Part model, mm, in its own coordinate system. A direction names the side the tool comes from. Round coordinates to 2 decimals unless told otherwise and drop trailing zeros. Write each loop counter-clockwise with the first axis right and the second up, starting at its lowest first coordinate (ties: lowest second). Pieces come first, ordered by that corner, then holes. Notation, with made-up numbers: (25, 51) -> (47, 51) arc R21 ccw to (47, 79) -> close; hole circle Ø5 at (-38.5, 17.25). An arc over 180 degrees is marked (long way). Return JSON: item names as keys, results as strings. Group by question number.
Solid Edge part; units mm, degrees
sketch "Sketch1" plane through (0, 0, 0) normal (1, 0, 0) x (0, 1, 0)
  line L0 (42, -40) -> (42, 40)
  line L1 (42, 40) -> (-42, 40)
  line L2 (-42, 40) -> (-42, -40)
  line L3 (-42, -40) -> (42, -40)
extrude "Protrusion1" add sketch "Sketch1" along normal blind 2
sketch "Sketch2" plane through (0, 0, 0) normal (1, 0, 0) x (0, 1, 0)
  line L0 (-42, 38) -> (-25, 38)
  line L1 (-25, 38) -> (-25, 40)
  line L2 (-25, 40) -> (-42, 40)
  line L3 (-42, 40) -> (-42, 38)
  line L4 (-15, 38) -> (-5, 38)
  line L5 (-5, 38) -> (-5, 40)
  line L6 (-5, 40) -> (-15, 40)
  line L7 (-15, 40) -> (-15, 38)
  line L8 (5, 38) -> (15, 38)
  line L9 (15, 38) -> (15, 40)
  line L10 (15, 40) -> (5, 40)
  line L11 (5, 40) -> (5, 38)
  line L12 (25, 38) -> (42, 38)
  line L13 (42, 38) -> (42, 40)
  line L14 (42, 40) -> (25, 40)
  line L15 (25, 40) -> (25, 38)
  line L16 (40, 15) -> (40, 25)
  line L17 (40, 25) -> (38, 25)
  line L18 (38, 25) -> (38, 15)
  line L19 (38, 15) -> (40, 15)
  line L20 (38, 5) -> (38, -5)
  line L21 (38, -5) -> (40, -5)
  line L22 (40, -5) -> (40, 5)
  line L23 (40, 5) -> (38, 5)
  line L24 (38, -15) -> (38, -25)
  line L25 (38, -25) -> (40, -25)
  line L26 (40, -25) -> (40, -15)
  line L27 (40, -15) -> (38, -15)
  line L28 (42, -38) -> (25, -38)
  line L29 (25, -38) -> (25, -40)
  line L30 (25, -40) -> (42, -40)
  line L31 (42, -40) -> (42, -38)
  line L32 (15, -38) -> (5, -38)
  line L33 (5, -38) -> (5, -40)
  line L34 (5, -40) -> (15, -40)
  line L35 (15, -40) -> (15, -38)
  line L36 (-5, -38) -> (-15, -38)
  line L37 (-15, -38) -> (-15, -40)
  line L38 (-15, -40) -> (-5, -40)
  line L39 (-5, -40) -> (-5, -38)
  line L40 (-25, -38) -> (-42, -38)
  line L41 (-42, -38) -> (-42, -40)
  line L42 (-42, -40) -> (-25, -40)
  line L43 (-25, -40) -> (-25, -38)
  line L44 (-38, -25) -> (-38, -15)
  line L45 (-38, -15) -> (-40, -15)
  line L46 (-40, -15) -> (-40, -25)
  line L47 (-40, -25) -> (-38, -25)
  line L48 (-38, -5) -> (-38, 5)
  line L49 (-38, 5) -> (-40, 5)
  line L50 (-40, 5) -> (-40, -5)
  line L51 (-40, -5) -> (-38, -5)
  line L52 (-38, 15) -> (-38, 25)
  line L53 (-38, 25) -> (-40, 25)
  line L54 (-40, 25) -> (-40, 15)
  line L55 (-40, 15) -> (-38, 15)
extrude "ExtrudedCutout_29" cut sketch "Sketch2" along normal blind 2
sketch "Sketch3" plane through (0, 0, 0) normal (1, 0, 0) x (0, 1, 0)
  line L0 (30, 15) -> (-30, 15)
  line L1 (-30, 15) -> (-30, -15)
  line L2 (-30, -15) -> (30, -15)
  line L3 (30, -15) -> (30, 15)
extrude "ExtrudedCutout_30" cut sketch "Sketch3" along normal blind 2
sketch "Sketch4" plane through (0, 0, 0) normal (1, 0, 0) x (0, 1, 0)
  circle A0 centre (0, 20) radius 2.25
  circle A1 centre (0, -20) radius 2.25
extrude "ExtrudedCutout_31" cut sketch "Sketch4" along normal blind 2
fillet "Round_1" radius 1 4 edges at (1, -42, -38) (1, 42, -38) (1, 42, 38) (1, -42, 38)
properties material "Acrylic, high impact grade"
Item 1: Cut at D-D (y = 0). Write the cut outline in (x, z), then the cut area to 3 significant figures.
Item 2: Two-plate mould, pull along Z, no slides. Class faces 1 (the face through (1, 33, 38)), 2 (the face through (1, -20, -40)), 3 (the face through (1, 39, -15)), 4 (the face through (0.986, -0.488, 22.196)): released by +Z, released by -Z, zero draft, split by the parting line, or undercut.
Item 3: Which spindle directions (+Z, -Z, +X, -X, +Y, -Y) get a long thin tool onto all of the face, cutting with end or side? Do faces 5 (the face through (1, 5, 39)), 6 (the face through (1, 25, 39)), 7 (the face through (1, 10, -38)), 8 (the face through (1, 38, 20)). Say none if no direction does.
Item 4: Cut at C-C (z = 20). Write the cut outline in (x, y).
Item 5: Wall check: L1, parallel to Z at x = 0.55, y = 39.5; L2, parallel to Z at x = 1, y = 0; L3, parallel to Z at x = 1.95, y = -21.5. Give the ranges that are in metal, low to high.
Item 6: Cut at A-A (z = 9). Write the cut outline in (x, y), then the cut area to 3 significant figures.
Item 7: Cut at B-B (y = 20). Write the cut outline in (x, z).
Item 8: Flat gauge pins, fed straight in: P1, Ø0.6, axis at x = 1.5, z = 39.5, coming from the +Y side; P2, Ø1, axis at x = 0.5, y = -38.5, coming from the -Z side; P3, Ø8, axis at y = 30, z = -28.5, coming from the -X side; P4, Ø1, axis at x = 0.5, y = 39.5, coming from the +Z side. Where does each tip first touch, or does it go through?
Checks:
{
 "1": {"outline": "(0, -40) -> (2, -40) -> (2, -22.25) -> (0, -22.25) -> close; (0, -17.75) -> (2, -17.75) -> (2, -15) -> (0, -15) -> close; (0, 15) -> (2, 15) -> (2, 17.75) -> (0, 17.75) -> close; (0, 22.25) -> (2, 22.25) -> (2, 40) -> (0, 40) -> close", "area": "82.0 mm2"},
 "2": {"face 1": "released by +Z", "face 2": "released by -Z", "face 3": "undercut", "face 4": "undercut"},
 "3": {"face 5": "+Z, +X, -X", "face 6": "+Z, +X, -X, +Y", "face 7": "-Z, +X, -X", "face 8": "+X, -X"},
 "4": {"outline": "(0, -42) -> (2, -42) -> (2, -40) -> (0, -40) -> close; (0, -38) -> (2, -38) -> (2, -2.25) -> (0, -2.25) -> close; (0, 2.25) -> (2, 2.25) -> (2, 38) -> (0, 38) -> close; (0, 40) -> (2, 40) -> (2, 42) -> (0, 42) -> close"},
 "5": {"L1": "z = -38 to -25, -15 to -5, 5 to 15, 25 to 38", "L2": "z = -40 to -22.25, -17.75 to -15, 15 to 17.75, 22.25 to 40", "L3": "z = -40 to -15, 15 to 40"},
 "6": {"outline": "(0, -42) -> (2, -42) -> (2, -30) -> (0, -30) -> close; (0, 30) -> (2, 30) -> (2, 42) -> (0, 42) -> close", "area": "48.0 mm2"},
 "7": {"outline": "(0, -40) -> (2, -40) -> (2, -15) -> (0, -15) -> close; (0, 15) -> (2, 15) -> (2, 40) -> (0, 40) -> close"},
 "8": {"P1": "stops at y = 25", "P2": "stops at z = -38", "P3": "stops at x = 0", "P4": "stops at z = 38"}
}
